CAD build for the part. Positions are in the model's coordinates, mm. A direction names the side the tool comes from. Give positions to 0.01 mm unless a question says otherwise; leave off trailing zeros. Order: outer loops, then holes, each group sorted by start corner. A loop starts at its lowest first (then second) coordinate and runs counter-clockwise, first axis right, second up.
Item 1: Band-saw the part on A-A on x = 0. Give the cut face in (y, z), plus the area to 3 significant figures.
Item 2: Which spindle directions (+Z, -Z, +X, -X, +Y, -Y) get a long thin tool onto all of the face, cutting with end or side? Do faces 1 (the flat face through (2, -2, 3)), 2 (the cylindrical face through (-1.08, -4.88, 2.49)). Say none if no direction does.
Item 3: Flat gauge pins, fed straight in: P1, Ø4, axis at x = 0, y = 3, coming from the -Z side; P2, Ø5, axis at y = -2, z = 15, coming from the -X side; P3, Ø1.5, axis at y = -1.5, z = 15.5, coming from the -X side; P4, Ø3, axis at x = 0, z = 22.5, coming from the -Y side. Where does each tip first touch, or does it go through?
Item 4: Band-saw the part on C-C on z = 10.5. Give the cut face in (x, y), plus the area to 3 significant figures.
Item 5: Wall check: L1, parallel to Y at x = -4, z = 2.25; L2, parallel to X at y = 1, z = 11.5; L3, parallel to Y at x = -1.25, z = 10.25. Give the ranges that are in metal, low to high.
```python
from build123d import *

# Parameters (mm, degrees)
SKETCH_R     = 5
PAD_DEPTH    = 3
SKETCH001_R  = 2.5
PAD001_DEPTH = 25
FILLET_R     = 2


with BuildPart() as part:
    # Sketch → Pad (new body)
    with BuildSketch(Plane.XY):
        Circle(SKETCH_R)
    extrude(amount=PAD_DEPTH)

    # Sketch001 → Pad001 (new body)
    with BuildSketch(Plane.XY.offset(3)):
        Circle(SKETCH001_R)
    extrude(amount=PAD001_DEPTH)

    # Fillet
    fillet_edges = [part.edges().sort_by_distance(p)[0] for p in [
        (-5, 0, 0),
    ]]
    fillet(fillet_edges, radius=FILLET_R)


solid = part.part
```
The answers:
1. outline: (-5, 2) arc R2 ccw to (-3, 0) - (3, 0) arc R2 ccw to (5, 2) - (5, 3) - (2.5, 3) - (2.5, 28) - (-2.5, 28) - (-2.5, 3) - (-5, 3) - close
1. area: 153 mm2
2. face 1: +Z
2. face 2: +Z, -Z
3. P1: stops at z = 0
3. P2: stops at x = -2.5
3. P3: stops at x = -2.38
3. P4: stops at y = -2.5
4. outline: circle Ø5 at (0, 0)
4. area: 19.6 mm2
5. L1: y = -3 to 3
5. L2: x = -2.29 to 2.29
5. L3: y = -2.17 to 2.17
